Build history of the part. All positions in model axes, mm. Face numbers are marked on the shaded views. A direction names the side the tool comes from. Round coordinates to 2 decimals unless told otherwise and drop trailing zeros. Write each loop counter-clockwise with the first axis right and the second up, starting at its lowest first coordinate (ties: lowest second). Pieces come first, ordered by that corner, then holes. Notation, with made-up numbers: (-36.5, 71.25) -> (11.5, 71.25) arc R36 cw to (11.5, 109.25) -> close; hole circle Ø10 at (-21.75, 23.25). An arc over 180 degrees is marked (long way). Return JSON: item names as keys, results as strings.
from build123d import *

# Parameters (mm, degrees)
SKETCH_1_R      = 4
SKETCH_1_R_2    = 1.55
EXTRUDE_1_DEPTH = 4
FILLET_1_R      = 2
FILLET_2_R      = 2


with BuildPart() as part:
    # 草图1 → 凸台-拉伸1 (new body)
    # profile 1 of 8: a face of its own
    with BuildSketch(Plane.XY):
        with BuildLine():
            ThreePointArc((-3.733382425, -1.435916317), (-3.830813532, 1.151028966), (-2.323665602, 3.25585291))
            Line((-2.323665602, 3.25585291), (-4.54302561, 9.026188932))
            ThreePointArc((-4.54302561, 9.026188932), (-7.072182387, 9.578587988), (-8.733382425, 11.564083683))
            Line((-8.733382425, 11.564083683), (-3.733382425, -1.435916317))
        make_face()
    # profile 2 of 8: a face of its own
    with BuildSketch(Plane.XY):
        with BuildLine():
            Line((4.54302561, 9.026188932), (2.323665602, 3.25585291))
            ThreePointArc((2.323665602, 3.25585291), (3.556308649, 1.831029436), (4, 0))
            ThreePointArc((4, 0), (3.932780804, -0.730229519), (3.733382425, -1.435916317))
            Line((3.733382425, -1.435916317), (8.733382425, 11.564083683))
            ThreePointArc((8.733382425, 11.564083683), (7.072182387, 9.578587988), (4.54302561, 9.026188932))
        make_face()
    # profile 3 of 8: a face of its own
    with BuildSketch(Plane.XY):
        with Locations((5, 13)):
            Circle(SKETCH_1_R)
        with Locations((5, 13)):
            Circle(SKETCH_1_R_2, mode=Mode.SUBTRACT)
    # profile 4 of 8: a face of its own
    with BuildSketch(Plane.XY):
        with Locations((-5, 13)):
            Circle(SKETCH_1_R)
        with Locations((-5, 13)):
            Circle(SKETCH_1_R_2, mode=Mode.SUBTRACT)
    # profile 5 of 8: a face of its own
    with BuildSketch(Plane.XY):
        with BuildLine():
            Line((-1, 13), (0, 13))
            Line((0, 13), (0, 17))
            Line((0, 17), (-5, 17))
            ThreePointArc((-5, 17), (-2.171572875, 15.828427125), (-1, 13))
        make_face()
    # profile 6 of 8: a face of its own
    with BuildSketch(Plane.XY):
        with BuildLine():
            Line((0, 17), (0, 13))
            Line((0, 13), (1, 13))
            ThreePointArc((1, 13), (2.171572875, 15.828427125), (5, 17))
            Line((5, 17), (0, 17))
        make_face()
    # profile 7 of 8: a face of its own
    with BuildSketch(Plane.XY):
        with BuildLine():
            ThreePointArc((2.323665602, 3.25585291), (1.219956631, 3.809423292), (0, 4))
            ThreePointArc((0, 4), (-1.219956631, 3.809423292), (-2.323665602, 3.25585291))
            ThreePointArc((-2.323665602, 3.25585291), (-3.830813532, 1.151028966), (-3.733382425, -1.435916317))
            ThreePointArc((-3.733382425, -1.435916317), (0, -4), (3.733382425, -1.435916317))
            ThreePointArc((3.733382425, -1.435916317), (3.932780804, -0.730229519), (4, 0))
            ThreePointArc((4, 0), (3.556308649, 1.831029436), (2.323665602, 3.25585291))
        make_face()
        with BuildLine():
            ThreePointArc((1.55, 0), (-1.096015511, -1.096015511), (0, 1.55))
            ThreePointArc((0, 1.55), (1.096015511, 1.096015511), (1.55, 0))
        make_face(mode=Mode.SUBTRACT)
    # profile 8 of 8: a face of its own
    with BuildSketch(Plane.XY):
        with BuildLine():
            ThreePointArc((2.323665602, 3.25585291), (1.219956631, 3.809423292), (0, 4))
            ThreePointArc((0, 4), (-1.219956631, 3.809423292), (-2.323665602, 3.25585291))
            ThreePointArc((-2.323665602, 3.25585291), (-3.830813532, 1.151028966), (-3.733382425, -1.435916317))
            ThreePointArc((-3.733382425, -1.435916317), (0, -4), (3.733382425, -1.435916317))
            ThreePointArc((3.733382425, -1.435916317), (3.932780804, -0.730229519), (4, 0))
            ThreePointArc((4, 0), (3.556308649, 1.831029436), (2.323665602, 3.25585291))
        make_face()
        with BuildLine():
            ThreePointArc((1.55, 0), (-1.096015511, -1.096015511), (0, 1.55))
            ThreePointArc((0, 1.55), (1.096015511, 1.096015511), (1.55, 0))
        make_face(mode=Mode.SUBTRACT)
    extrude(amount=EXTRUDE_1_DEPTH)

    # 圆角1
    # the kernel refuses this fillet: 2 mm, written as the material it adds along each edge
    with BuildSketch(Plane(origin=(-4.54302561, 9.026188932, 0), x_dir=(0.9477918493687586, 0.3188896521841818, 0), z_dir=(0, 0, 1))) as fillet_1_piece_1:
        with BuildLine():
            CenterArc((2.085226569, -1.956035073), FILLET_1_R, 102.035790206, 80.405931773)
            Line((0.087042425, -2.041241452), (0, 0))
            ThreePointArc((0, 0), (0.834090628, -0.087929854), (1.668181255, 0))
        make_face()
    extrude(amount=4)
    with BuildSketch(Plane(origin=(-2.323665602, 3.25585291, 0), x_dir=(-0.3589790793088693, 0.9333456062030594, 0), z_dir=(0, 0, 1)), Plane(origin=(4.54302561, 9.026188932, 0), x_dir=(-0.3589790793088692, -0.9333456062030594, 0), z_dir=(0, 0, 1))) as fillet_1_piece_2:
        with BuildLine():
            CenterArc((2.043096437, -2), FILLET_1_R, 90, 80.405931773)
            ThreePointArc((0.071069843, -1.666666667), (0.123384942, -0.829587241), (0, 0))
            Line((0, 0), (2.043096437, 0))
        make_face()
    extrude(amount=4)
    with BuildSketch(Plane(origin=(2.323665602, 3.25585291, 0), x_dir=(0.35897907930886913, 0.9333456062030596, 0), z_dir=(0, 0, 1))) as fillet_1_piece_3:
        with BuildLine():
            CenterArc((2.043096437, 2), FILLET_1_R, 189.594068227, 80.405931773)
            ThreePointArc((0.071069843, 1.666666667), (0.123384942, 0.829587241), (0, 0))
            Line((0, 0), (2.043096437, 0))
        make_face()
    extrude(amount=4)
    with BuildSketch(Plane(origin=(1, 13, 0), x_dir=(-1, 0, 0), z_dir=(0, 0, 1))) as fillet_1_piece_4:
        with BuildLine():
            CenterArc((1.656854249, 2), FILLET_1_R, 199.471220634, 70.528779366)
            ThreePointArc((-0.228763834, 1.333333333), (-0.057605761, 0.676407915), (0, 0))
            Line((0, 0), (1.656854249, 0))
        make_face()
    extrude(amount=4)
    with BuildSketch(Plane(origin=(-1, 13, 0), x_dir=(-0.16910197872576255, -0.9855985596534887, 0), z_dir=(0, 0, 1))) as fillet_1_piece_5:
        with BuildLine():
            CenterArc((1.691019787, 1.971197119), FILLET_1_R, 189.735610317, 70.528779366)
            Line((-0.280177332, 1.632993162), (0, 0))
            ThreePointArc((0, 0), (0.676407915, 0.057605761), (1.35281583, 0))
        make_face()
    extrude(amount=4)

    # 圆角2
    fillet_2_edges = [part.edges().sort_by_distance(p)[0] for p in [
        (0, 12.889058627, 2),
    ]]
    fillet(fillet_2_edges, radius=FILLET_2_R)


solid = part.part
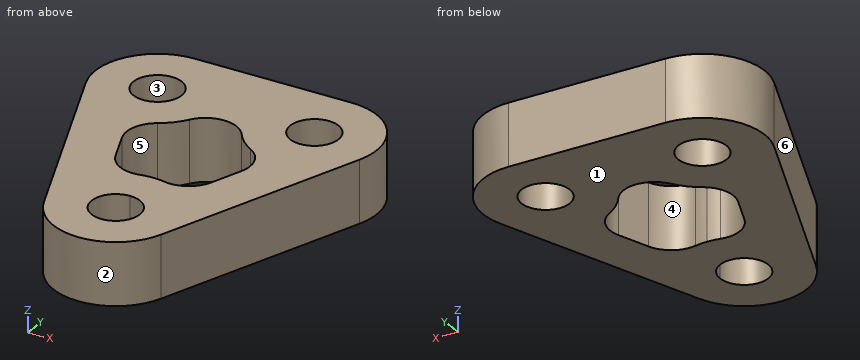
Q1. Wall check: L1, parallel to X at y = 13.25, z = 2.35; L2, parallel to Y at x = -0.5, z = 0.35; L3, parallel to Y at x = 2, z = 1.6. Give the ranges that are in metal, low to high.
Verdict:
{"L1": "x = -8.99 to -6.53, -3.47 to 3.47, 6.53 to 8.99", "L2": "y = -3.97 to -1.47, 1.47 to 3.97, 11.62 to 17", "L3": "y = -3.46 to 4.05, 10.35 to 17"}
Q2. 3-axis set-ups, long thin cutter, end or side, ignore diameter. For the marked faces 5 and 6: which of +Z, -Z, +X, -X, +Y, -Y reach the whole face in a straight line?
Verdict:
{"face 5": "+Z, -Z", "face 6": "+Z, -Z, -X, -Y"}
Q3. Saw through at D-D on z = 0.8. Count the separate pieces of the cut face and the enclosed holes in it, then the cut area to 3 significant figures.
Verdict:
{"separate pieces": "1", "enclosed holes": "4", "area": "199 mm²"}
Q4. Pin check, flat tips, straight feed: pin 1 Ø1.9 at (x, y) = (0, 0) entering from -Z; pin 2 Ø2 at (y, z) = (15, 1) entering from -X. Stop position of each tip, or through.
Verdict:
{"pin 1": "passes through", "pin 2": "stops at x = -8.87"}
Q5. Saw through at C-C on y = 8.5. List the corners of the cut face in (x, z), then the cut area to 3 significant figures.
Verdict:
{"outline": "(-7.55, 0) -> (-3.83, 0) -> (-3.83, 4) -> (-7.55, 4) -> close; (3.83, 0) -> (7.55, 0) -> (7.55, 4) -> (3.83, 4) -> close", "area": "29.8 mm²"}
Q6. Saw through at A-A on y = 13. List the corners of the cut face in (x, z), then the cut area to 3 significant figures.
Verdict:
{"outline": "(-9, 0) -> (-6.55, 0) -> (-6.55, 4) -> (-9, 4) -> close; (-3.45, 0) -> (3.45, 0) -> (3.45, 4) -> (-3.45, 4) -> close; (6.55, 0) -> (9, 0) -> (9, 4) -> (6.55, 4) -> close", "area": "47.2 mm²"}
Q7. Two-plate mould, pull along X, no slides. Class the marked faces 1, 2, 3 and 4: +X half, -X half, draft (parallel to the pull), parting line (faces both ways), or undercut.
Verdict:
{"face 1": "draft", "face 2": "parting line", "face 3": "undercut", "face 4": "undercut"}
Q8. Saw through at B-B on x = -5.75. List the corners of the cut face in (y, z), then the cut area to 3 significant figures.
Verdict:
{"outline": "(3.81, 0) -> (11.64, 0) -> (11.64, 4) -> (3.81, 4) -> close; (14.36, 0) -> (16.93, 0) -> (16.93, 4) -> (14.36, 4) -> close", "area": "41.6 mm²"}
